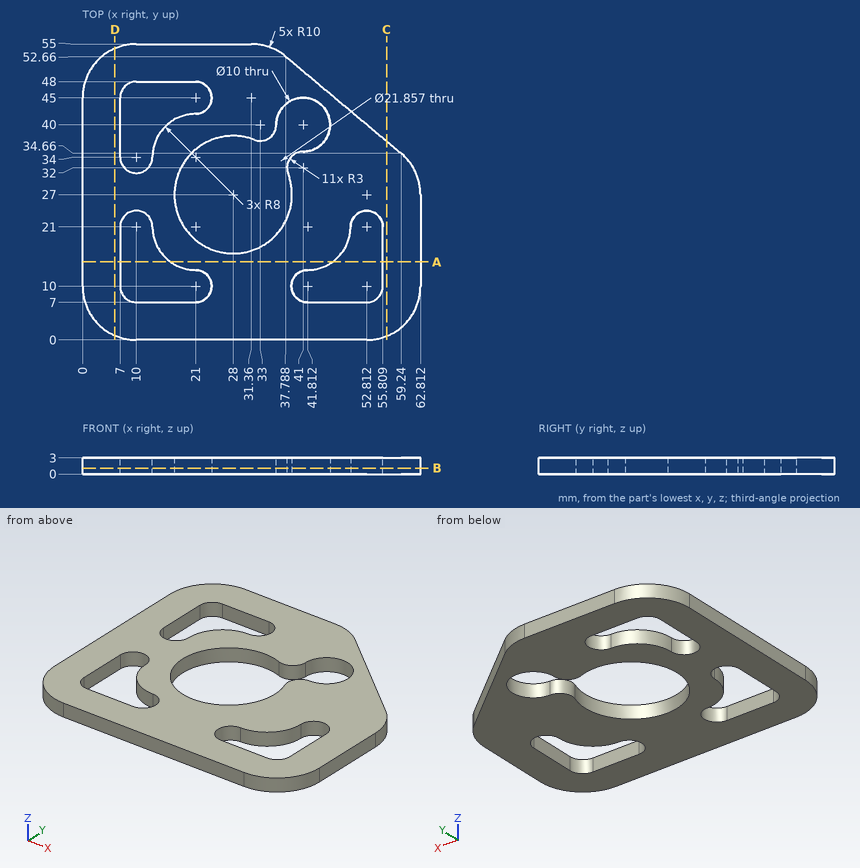
For this review, use the dimensioned drawing (mm, ordinates from the lowest corner) and the shaded views. Coordinates: 2 decimals unless noted, no trailing zeros. Loops run counter-clockwise (first coordinate to the right, second up) from the corner with the lowest first, then second, coordinate; pieces in that order, holes last.
1. Add section D-D, the plane x = 6. Give the boundary of the cut face in (y, z) (1 decimal), then the cut area to 3 significant figures.
2. For line 1 (Y direction, x = 43, z = 0.35); line 2 (X direction, y = 27, z = 1.45); line 3 (Y direction, x = 28, z = 1.4), list the stretches that pass through material, from the lowest coordinate up.
3. Add section A-A, the plane y = 14.5. Give the boundary of the cut face in (x, z) (1 decimal).
4. Insertion check: P1, Ø1.5, axis at x = 43.5, z = 2.5, coming from the +Y side; P2, Ø9, axis at x = 41, y = 40, coming from the +Z side. Each pin has a flat end and moves straight along its axis. Give the tip position at first contact, or say it passes through.
5. Add section C-C, the plane x = 56.5. Give the boundary of the cut face in (y, z) (1 decimal), then the cut area to 3 significant figures.
6. Add section B-B, the plane z = 1.1. Count the separate pieces of the cut face and the enclosed holes in it, then the cut area to 3 significant figures.
Result:
1. outline: (0.8, 0) - (54.2, 0) - (54.2, 3) - (0.8, 3) - close
1. area: 160 mm2
2. line 1: y = 0 to 7, 13.09 to 35.42, 44.58 to 48.29
2. line 2: x = 0 to 17.07, 38.93 to 62.81
2. line 3: y = 0 to 16.07, 37.93 to 55
3. outline: (0, 0) - (7, 0) - (7, 3) - (0, 3) - close; (16.3, 0) - (46.5, 0) - (46.5, 3) - (16.3, 3) - close; (55.8, 0) - (62.8, 0) - (62.8, 3) - (55.8, 3) - close
4. P1: stops at y = 48.5
4. P2: passes through
5. outline: (0.7, 0) - (37, 0) - (37, 3) - (0.7, 3) - close
5. area: 109 mm2
6. separate pieces: 1
6. enclosed holes: 4
6. area: 2,070 mm2
